The listing builds one solid part. Answer for the finished solid, in the listing's coordinates (mm). A direction names the side the tool comes from. Give positions to 0.01 mm unless a question says otherwise; leave off trailing zeros. Loops run counter-clockwise (first coordinate to the right, second up) from the corner with the lowest first, then second, coordinate; pieces in that order, holes last. Notation, with made-up numbers: (69, 60) - (96, 60) arc R28 cw to (96, 91) - close; hole circle Ø7 at (45, 44). An arc over 180 degrees is marked (long way). Answer in a Markdown table with one row per item. Add a question column.
```python
from build123d import *

# Parameters (mm, degrees)
ESQUISSE1_W             = 12
ESQUISSE1_H             = 12
BOSS_EXTRU_1_DEPTH      = 2
ESQUISSE2_R             = 5
BOSS_EXTRU_2_DEPTH      = 2
ESQUISSE3_R             = 2.5
ENL_V_MAT_EXTRU_1_DEPTH = 2


with BuildPart() as part:
    # Esquisse1 → Boss.-Extru.1 (new body)
    with BuildSketch(Plane.XY):
        with BuildLine():
            Line((16.5, 6), (6, 6))
            Line((6, 6), (6, -6))
            Line((6, -6), (16.5, -6))
            ThreePointArc((16.5, -6), (22.5, 0), (16.5, 6))
        make_face()
        Rectangle(ESQUISSE1_W, ESQUISSE1_H)
        with BuildLine():
            Line((-6, 15), (-6, 6))
            Line((-6, 6), (6, 6))
            Line((6, 6), (6, 15))
            ThreePointArc((6, 15), (0, 21), (-6, 15))
        make_face()
        with BuildLine():
            Line((-6, 6), (-16.5, 6))
            ThreePointArc((-16.5, 6), (-22.5, 0), (-16.5, -6))
            Line((-16.5, -6), (-6, -6))
            Line((-6, -6), (-6, 6))
        make_face()
        with BuildLine():
            Line((6, -6), (-6, -6))
            Line((-6, -6), (-6, -15))
            ThreePointArc((-6, -15), (0, -21), (6, -15))
            Line((6, -15), (6, -6))
        make_face()
    extrude(amount=BOSS_EXTRU_1_DEPTH)

    # Esquisse2 → Boss.-Extru.2 (add)
    with BuildSketch(Plane(origin=(0, 0, 0), x_dir=(-1, 0, 0), z_dir=(0, 0, -1))):
        with Locations(Location((0, 0, 0), (0, 0, 180))):
            Circle(ESQUISSE2_R)
    extrude(amount=BOSS_EXTRU_2_DEPTH)

    # Esquisse3 → Enlèv. mat.-Extru.1 (cut)
    with BuildSketch(Plane(origin=(0, 0, -2), x_dir=(-1, 0, 0), z_dir=(0, 0, -1))):
        Circle(ESQUISSE3_R)
    extrude(amount=-ENL_V_MAT_EXTRU_1_DEPTH, mode=Mode.SUBTRACT)


solid = part.part
```
(1) A tool of negligible diameter and unlimited length cuts with its end or side. For faces 1 (the face through (11, 6, 1)), 2 (the face through (-11, 6, 1)), 3 (the face through (-6, -10, 1)), 4 (the face through (11, -6, 1)), 5 (the face through (-5, 0, -1)), from which of +Z, -Z, +X, -X, +Y, -Y can it reach the whole face along a straight path? Write none if from no direction.
(2) A cutting plane is placed at A-A on z = -0.5. Determine the outline of the cut face in (x, y), plus the area to 3 significant figures.
(3) A cutting plane is placed at B-B on x = 0. Determine the outline of the cut face in (y, z).
(4) A cutting plane is placed at D-D on y = -6.5. Determine the outline of the cut face in (x, z), plus the area to 3 significant figures.
(5) Given pin 1 Ø2 at (y, z) = (12, 0.5) entering from +X; pin 2 Ø2 at (x, z) = (12.5, 0.5) entering from -Y; pin 3 Ø1 at (y, z) = (-9.5, 1) entering from -X; pin 4 Ø4 at (x, y) = (-1, -0.5) entering from -Z, each flat-ended and moving along its own axis, determine where each tip first touches the part or whether it passes through.
(6) The mould has two halves that part along X. Classify faces 6 (the face through (0, 0, 2)), 7 (the face through (0, 0, 0)), 8 (the face through (6, 10, 1)): pulls with the +X half, pulls with the -X half, needs draft (parallel to the pull), parting line crosses it, or undercut.
(7) A cutting plane is placed at C-C on y = 0. Determine the outline of the cut face in (x, z).
(8) Find the intervals of material crossed by line 1 along Y through (x, z) = (0, -1.45); line 2 along X through (y, z) = (8.5, 0.7), in increasing order. Write a range as [from, to].
Evaluation:
| question | item | result |
|---|---|---|
| 1 | face 1 | +Z, -Z, +X, +Y |
| 1 | face 2 | +Z, -Z, -X, +Y |
| 1 | face 3 | +Z, -Z, -X, -Y |
| 1 | face 4 | +Z, -Z, +X, -Y |
| 1 | face 5 | -Z |
| 2 | outline | circle Ø10 at (0, 0); hole circle Ø5 at (0, 0) |
| 2 | area | 58.9 mm² |
| 3 | outline | (-21, 0) - (-5, 0) - (-5, -2) - (-2.5, -2) - (-2.5, 0) - (2.5, 0) - (2.5, -2) - (5, -2) - (5, 0) - (21, 0) - (21, 2) - (-21, 2) - close |
| 4 | outline | (-6, 0) - (6, 0) - (6, 2) - (-6, 2) - close |
| 4 | area | 24.0 mm² |
| 5 | pin 1 | stops at x = 6 |
| 5 | pin 2 | stops at y = -6 |
| 5 | pin 3 | stops at x = -6 |
| 5 | pin 4 | stops at z = -2 |
| 6 | face 6 | needs draft |
| 6 | face 7 | undercut |
| 6 | face 8 | pulls with the +X half |
| 7 | outline | (-22.5, 0) - (-5, 0) - (-5, -2) - (-2.5, -2) - (-2.5, 0) - (2.5, 0) - (2.5, -2) - (5, -2) - (5, 0) - (22.5, 0) - (22.5, 2) - (-22.5, 2) - close |
| 8 | line 1 | y = [-5, -2.5], [2.5, 5] |
| 8 | line 2 | x = [-6, 6] |
